Build history of the part. All positions in model axes, mm. A direction names the side the tool comes from. Round coordinates to 2 decimals unless told otherwise and drop trailing zeros. Loops run counter-clockwise (first coordinate to the right, second up) from the corner with the lowest first, then second, coordinate; pieces in that order, holes last. Notation, with made-up numbers: (-11.75, 48) - (39.25, 48) arc R24 cw to (39.25, 82) - close; hole circle Ø3 at (77.25, 55). An arc over 180 degrees is marked (long way). Answer as CSV lines item,"result". Start each with the question number.
```python
from build123d import *

# Parameters (mm, degrees)
F0_W      = 130
F0_H      = 248
F1_DEPTH  = 205
F2_W      = 94.3407235295
F2_H      = 248
F2_R      = 9
F2_W_2    = 73.0899348855
F2_H_2    = 49.802608788
F3_DEPTH  = 2
F4_W      = 130
F4_H      = 10
F5_DEPTH  = 20
F7_DEPTH  = 10
F9_DEPTH  = 130.001
F10_F1_R  = 1
F10_F2_R  = 1
F11_DEPTH = 18


with BuildPart() as f1:
    # F0 (on Front) → F1 (new body)
    with BuildSketch(Plane.XZ):
        Rectangle(F0_W, F0_H)
    extrude(amount=F1_DEPTH)

    # F2 (on face) → F3 (cut)
    with BuildSketch(Plane.XZ.offset(205)):
        with Locations((17.8296382353, 0)):
            Rectangle(F2_W, F2_H)
        with BuildLine():
            ThreePointArc((-4.041418053, 4.0888261301), (-10.3760691988, 21.9367014989), (-4.1207936375, 39.8125507927))
            Line((-4.1207936375, 39.8125507927), (4.0327052851, 31.6590518702))
            ThreePointArc((4.0327052851, 31.6590518702), (1.0381912146, 21.9360306033), (4.1054760852, 12.2357202683))
            Line((4.1054760852, 12.2357202683), (-4.041418053, 4.0888261301))
        make_face(mode=Mode.SUBTRACT)
        with BuildLine():
            Line((27.7718433373, 7.9199138179), (35.9253422598, -0.2335851046))
            ThreePointArc((35.9253422598, -0.2335851046), (18.0492121242, -6.4888600406), (0.2011808104, -0.1538563808))
            Line((0.2011808104, -0.1538563808), (8.3480462814, 7.9930090903))
            ThreePointArc((8.3480462814, 7.9930090903), (18.0485383783, 4.9254008127), (27.7718433373, 7.9199138179))
        make_face(mode=Mode.SUBTRACT)
        with Locations((18.1127931993, 22.0000017322)):
            Circle(F2_R, mode=Mode.SUBTRACT)
        with BuildLine():
            ThreePointArc((0.1029558919, 44.0740826376), (18.0492420298, 50.4888635717), (36.0239688015, 44.1542129845))
            Line((36.0239688015, 44.1542129845), (27.8770746633, 36.0073188463))
            ThreePointArc((27.8770746633, 36.0073188463), (18.0486241947, 39.0746029744), (8.2435056862, 35.9335328433))
            Line((8.2435056862, 35.9335328433), (0.1029558919, 44.0740826376))
        make_face(mode=Mode.SUBTRACT)
        with BuildLine():
            ThreePointArc((40.2666513123, 39.9116141211), (46.6016556639, 21.9367314045), (40.1868741048, 3.9901644247))
            Line((40.1868741048, 3.9901644247), (32.0463243105, 12.130714219))
            ThreePointArc((32.0463243105, 12.130714219), (35.1873955054, 21.9361164198), (32.1197858413, 31.7647486501))
            Line((32.1197858413, 31.7647486501), (40.2666513123, 39.9116141211))
        make_face(mode=Mode.SUBTRACT)
        with Locations((18.2467956167, 91.3970731086)):
            Rectangle(F2_W_2, F2_H_2, mode=Mode.SUBTRACT)
    extrude(amount=-F3_DEPTH, mode=Mode.SUBTRACT)

    # F4 (on face) → F5 (join)
    with BuildSketch(Plane(origin=(0, 0, 0), x_dir=(-1, 0, 0), z_dir=(0, 1, 0))):
        with Locations((0, 129)):
            Rectangle(F4_W, F4_H)
        with Locations((0, -129)):
            Rectangle(F4_W, F4_H)
    extrude(amount=-F5_DEPTH)

    # F6 (on face) → F7 (cut, through all)
    with BuildSketch(Plane.XY.offset(134)):
        Polygon((63, -2), (-63, -2), (-63, -20), (63, -20), (63, -18), align=None)
    extrude(amount=-F7_DEPTH, mode=Mode.SUBTRACT)

    # F8 (on face) → F9 (cut, through all)
    with BuildSketch(Plane.YZ.offset(65)):
        Polygon((-20, 134), (-20, 124), (-2, 134), align=None)
    extrude(amount=-F9_DEPTH, mode=Mode.SUBTRACT)

    # F10: fillet of radius 1 on 29 edges, made by hand

    # F10_f1
    f10_f1_edges = [f1.edges().sort_by_distance(p)[0] for p in [
        (-29.3407235295, -203, 0),
        (-0.0440441762, -203, 35.7358013315),
        (1.0381912146, -203, 21.9360306033),
        (0.0320290161, -203, 8.1622731992),
        (-10.3760691988, -203, 21.9367014989),
        (4.2746135459, -203, 3.9195763547),
        (18.0485383783, -203, 4.9254008127),
        (31.8485927986, -203, 3.8431643567),
        (18.0492121242, -203, -6.4888600406),
        (9.1127931993, -203, 22.0000017322),
        (18.0492420298, -203, 50.4888635717),
        (31.9505217324, -203, 40.0807659154),
        (18.0486241947, -203, 39.0746029744),
        (4.173230789, -203, 40.0038077405),
        (36.1932185768, -203, 35.8381813856),
        (46.6016556639, -203, 21.9367314045),
        (36.1165992076, -203, 8.0604393219),
        (35.1873955054, -203, 21.9361164198),
        (18.2467956167, -203, 66.4957687146),
        (-18.2981718261, -203, 91.3970731086),
        (18.2467956167, -203, 116.2983775027),
        (54.7917630594, -203, 91.3970731086),
    ]]
    fillet(f10_f1_edges, radius=F10_F1_R)

    # F10_f2
    f10_f2_edges = [f1.edges().sort_by_distance(p)[0] for p in [
        (-65, -112.5, 124),
        (-65, -11, 129),
        (65, -11, 129),
        (65, -111.5, 124),
        (18.3296382353, -203, 124),
        (18.3296382353, -203, -124),
        (65, -203, 0),
        (-29.0478303106, -203.2928932188, -124),
        (-29.0478303106, -203.2928932188, 124),
    ]]
    fillet(f10_f2_edges, radius=F10_F2_R)

    # F11 (cut): a face of the model
    f11_faces = [f1.faces().sort_by_distance(p)[0] for p in [
        (0, -20, -129),
    ]]
    extrude(f11_faces, amount=-F11_DEPTH, mode=Mode.SUBTRACT)


solid = f1.part
```
Q1. Band-saw the part on A-A, the plane x = -37.5. List the corners of the cut face in (y, z), then the cut area to 3 significant figures.
Q2. Pin check, flat tips, straight feed: pin 1 Ø0.8 at (x, y) = (30, -204.5) entering from -Z; pin 2 Ø8 at (x, z) = (-20.5, 127.5) entering from -Y; pin 3 Ø1.1 at (y, z) = (-204.5, 27.5) entering from +X. Stop position of each tip, or through.
Q3. Tool access for faces 1 (the flat face through (65, -100, -2)), 2 (the flat face through (1, -2, -129)), 3 (the flat face through (18, -205, 43)), 4 (the cylindrical face through (17.777, -204.507, 50.487)), 5 (the cylindrical face through (46.6, -204.5, 22.2)): list every direction of +Z, -Z, +X, -X, +Y, -Y with a clear straight run to the whole face (end or side of a thin tool).
Q4. Wall check: probe 1 along Y at (x, z) = (-9.5, 34.5); probe 2 along Z at (x, y) = (-55, -63.5). Give the ranges that are in metal, low to high. Write a range as [from, to].
Q5. Two-plate mould, pull along Z, no slides. Class faces 6 (the flat face through (1, 0, 2)), 7 (the cylindrical face through (0.096, -203.285, 7.801)), 8 (the flat face through (-63.49, -11.13, 128.93)): released by +Z, released by -Z, zero draft, split by the parting line, or undercut.
Q6. Band-saw the part on B-B, the plane y = -85. List the corners of the cut face in (x, z).
Reported:
1,outline,"(-205, -124) - (-2, -124) - (-2, -134) - (0, -134) - (0, 134) - (-2, 134) - (-2, 124) - (-205, 124) - close"
1,area,"50,900 mm2"
2,pin 1,"stops at z = -4.07"
2,pin 2,"stops at y = -202.87"
2,pin 3,"stops at x = 46.17"
3,face 1,"+Z, -Z, +X, +Y, -Y"
3,face 2,"-Z, +X, -X, -Y"
3,face 3,"+Z, -Z, +X, -X, -Y"
3,face 4,"-Y"
3,face 5,"+X, -Y"
4,probe 1,"y = [-203, 0]"
4,probe 2,"z = [-124, 124]"
5,face 6,"zero draft"
5,face 7,"undercut"
5,face 8,"released by +Z"
6,outline,"(-65, -124) - (65, -124) - (65, 123) arc R1 ccw to (64, 124) - (-64, 124) arc R1 ccw to (-65, 123) - close"
